Design review of the part built by this model. Coordinates are the model's own, in mm. A direction names the side the tool comes from. Give positions to 0.01 mm unless a question says otherwise; leave off trailing zeros. Write each loop counter-clockwise with the first axis right and the second up, starting at its lowest first coordinate (ties: lowest second). Pieces come first, ordered by that corner, then holes. Notation, with made-up numbers: (15, 35.25) -> (65, 35.25) arc R28 ccw to (65, 58.25) -> close; hole circle Ø7 at (-11, 88). An arc over 180 degrees is marked (long way). Put each result on its own line as item: value. Start each with the question number.
from build123d import *

# Parameters (mm, degrees)
SKETCH1_R           = 12
BOSS_EXTRUDE1_DEPTH = 10
SKETCH2_W           = 20
SKETCH2_H           = 40
BOSS_EXTRUDE2_DEPTH = 20
SKETCH3_W           = 20
SKETCH3_H           = 20
BOSS_EXTRUDE3_DEPTH = 7


with BuildPart() as part:
    # Sketch1 → Boss-Extrude1 (new body)
    with BuildSketch(Plane.XY):
        with BuildLine():
            Line((30, -20), (-30, -20))
            ThreePointArc((-30, -20), (-50, 0), (-30, 20))
            Line((-30, 20), (30, 20))
            Line((30, 20), (30, -20))
        make_face()
        with Locations((-30, 0)):
            Circle(SKETCH1_R, mode=Mode.SUBTRACT)
    extrude(amount=BOSS_EXTRUDE1_DEPTH)

    # Sketch2 → Boss-Extrude2 (add)
    with BuildSketch(Plane.XY.offset(10)):
        with Locations((20, 0)):
            Rectangle(SKETCH2_W, SKETCH2_H)
    extrude(amount=BOSS_EXTRUDE2_DEPTH)

    # Sketch3 → Boss-Extrude3 (add)
    with BuildSketch(Plane.XY.offset(30)):
        with Locations((20, 0)):
            Rectangle(SKETCH3_W, SKETCH3_H)
    extrude(amount=BOSS_EXTRUDE3_DEPTH)


solid = part.part
Q1. For pin 1 (12 mm diameter, centred on y = -9.5, z = 24.5, fed in from -X); pin 2 (11 mm diameter, centred on x = 15.5, y = 16.5, fed in from +Z); pin 3 (3.5 mm diameter, centred on x = 23.5, z = 34.5, fed in from -Y), all flat-tipped, find the tip position at first contact; note any pin that passes through.
Q2. Take a section at C-C on z = 7. Give the boundary of the cut face in (x, y), then the cut area to 3 significant figures.
Q3. Take a section at D-D on x = -27. Give the boundary of the cut face in (y, z).
Q4. To check wall thickness, follow probe 1 along Y at (x, z) = (-30, 8); probe 2 along X at (y, z) = (-11.5, 20); probe 3 along X at (y, z) = (-6, 2). State the ranges of each line that lie inside material, in increasing order. Write a range as from..to.
Q5. Take a section at B-B on x = 17. Give the boundary of the cut face in (y, z), then the cut area to 3 significant figures.
Q6. Mouldability with a two-part tool opening along Y and no side actions: class faces 1 (the face through (-50, 0, 5)), 2 (the face through (6, -20, 8)), 3 (the face through (-18.915, -4.596, 4.93)) as +Y half, -Y half, draft (parallel to the pull), parting line (faces both ways), or undercut.
Q7. Machinability: for faces 4 (the face through (20, -10, 33)), 5 (the face through (-13, 0, 10)), 6 (the face through (30, 0, 18)), 7 (the face through (20, 15, 30)), which of the approach directions +Z, -Z, +X, -X, +Y, -Y give a long, thin tool a straight path to every point of the face, cutting with its end or side? Answer none if there is none.
Q8. Take a section at A-A on y = 0. Give the boundary of the cut face in (x, z), then the cut area to 3 significant figures.
Result:
1. pin 1: stops at x = 10
1. pin 2: stops at z = 30
1. pin 3: stops at y = -10
2. outline: (-30, -20) -> (30, -20) -> (30, 20) -> (-30, 20) arc R20 ccw to start; hole circle Ø24 at (-30, 0)
2. area: 2,580 mm^2
3. outline: (-20, 0) -> (-11.62, 0) -> (-11.62, 10) -> (-20, 10) -> close; (11.62, 0) -> (20, 0) -> (20, 10) -> (11.62, 10) -> close
4. probe 1: y = -20..-12, 12..20
4. probe 2: x = 10..30
4. probe 3: x = -49.08..-40.39, -19.61..30
5. outline: (-20, 0) -> (20, 0) -> (20, 30) -> (10, 30) -> (10, 37) -> (-10, 37) -> (-10, 30) -> (-20, 30) -> close
5. area: 1,340 mm^2
6. face 1: parting line
6. face 2: -Y half
6. face 3: undercut
7. face 4: +Z, +X, -X, -Y
7. face 5: +Z, -X, +Y, -Y
7. face 6: +Z, -Z, +X, +Y, -Y
7. face 7: +Z, +X, -X, +Y
8. outline: (-50, 0) -> (-42, 0) -> (-42, 10) -> (-50, 10) -> close; (-18, 0) -> (30, 0) -> (30, 37) -> (10, 37) -> (10, 10) -> (-18, 10) -> close
8. area: 1,100 mm^2
